Read the model definition and answer for the solid it produces. Units are mm, in the model's axes. A direction names the side the tool comes from. Give positions to 0.01 mm unless a question says otherwise; leave off trailing zeros. Loops run counter-clockwise (first coordinate to the right, second up) from the corner with the lowest first, then second, coordinate; pieces in that order, holes last. Notation, with made-up numbers: (2.25, -10.5) - (51.25, -10.5) arc R16 ccw to (51.25, 20.5) - close; hole circle Ø2 at (-35.75, 76). An arc over 180 degrees is marked (long way). Use a Markdown table: item, result. Add a question column.
Item 1: A cutting plane is placed at C-C (x = 0). Determine the outline of the cut face in (y, z).
Item 2: For a pull along Z with two mould halves and no side action, classify faces 1 (the face through (-4, 15, -1)), 2 (the face through (3.3, 5.1, 2.2)), 3 (the face through (3.417, 4.558, 0.759)) as +Z half, -Z half, draft (parallel to the pull), parting line (faces both ways), or undercut.
Item 3: Each of these flat-tipped pins is pushed along its axis until it touches: P1, Ø3, axis at x = -1.5, y = 15.5, coming from the +Z side; P2, Ø1, axis at x = 3, y = 16, coming from the +Z side; P3, Ø1.5, axis at x = 4, y = 17, coming from the +Z side. Where does it stop, or does it pass through?
Item 4: A cutting plane is placed at A-A (y = 13.25). Determine the outline of the cut face in (x, z).
Item 5: Consider probe 1 along Z at (x, y) = (-1, 12.75); probe 2 along X at (y, z) = (11, -0.5); probe 3 along Z at (x, y) = (-4, 16.75). Determine where each line is inside the solid, lowest interval first. Write a range as [from, to].
Item 6: Which of the six approach directions +Z, -Z, +X, -X, +Y, -Y give full straight-line access (tool end or side, diameter ignored) to faces 4 (the face through (0.09, 16.16, -4.75)), 5 (the face through (2, 4, 2)), 6 (the face through (-0.09, 16.16, 4.75)), 7 (the face through (0, 14, -3))?
Item 7: A cutting plane is placed at B-B (z = 0). Determine the outline of the cut face in (x, y), plus the area to 3 significant figures.
Item 8: A cutting plane is placed at D-D (y = 6). Determine the outline of the cut face in (x, z).
from build123d import *

# Parameters (mm, degrees)
ENL_V_MAT_EXTRU_1_REACH             = 23.308
ESQUISSE2_W                         = 2
ESQUISSE2_H                         = 8
ENL_V_MAT_EXTRU_1_DIRECTION_2_REACH = 23.308


with BuildPart() as part:
    # Esquisse1 → Révolution1 (revolve)
    with BuildSketch(Plane.XY, mode=Mode.PRIVATE) as r_volution1_sk:
        with BuildLine():
            Line((0, 0), (-2.5, 0))
            Line((-2.5, 0), (-2.5, 4))
            Line((-2.5, 4), (-3.5, 4))
            Line((-3.5, 4), (-3.5, 5.1))
            Line((-3.5, 5.1), (-5, 5.1))
            Line((-5, 5.1), (-5, 12.1))
            Line((-5, 12.1), (-4.75, 12.1))
            Line((-4.75, 12.1), (-4.75, 20.1))
            Line((-4.75, 20.1), (-4.55, 20.1))
            Line((-4.55, 20.1), (-3, 16.1))
            Line((-3, 16.1), (-3, 12.1))
            ThreePointArc((-3, 12.1), (-2.121320344, 9.978679656), (0, 9.1))
            Line((0, 9.1), (0, 0))
        make_face()
    revolve(r_volution1_sk.sketch.rotate(Axis((0, -1.292585524, 0), (0, 1, 0)), 270), axis=Axis((0, -1.292585524, 0), (0, 1, 0)))

    # Esquisse2 → Enlèv. mat.-Extru.1 (cut, up to next)
    with BuildSketch(Plane(origin=(0, 0, 0), x_dir=(0, 0, -1), z_dir=(1, 0, 0)), mode=Mode.PRIVATE) as enl_v_mat_extru_1_sk1:
        with Locations((0, 16.1)):
            Rectangle(ESQUISSE2_W, ESQUISSE2_H)
    enl_v_mat_extru_1_tool1 = extrude(enl_v_mat_extru_1_sk1.sketch, amount=-ENL_V_MAT_EXTRU_1_REACH, mode=Mode.PRIVATE) & part.part
    add(enl_v_mat_extru_1_tool1.solids().sort_by_distance((0, 16.1, 0))[0], mode=Mode.SUBTRACT)

    # Esquisse2 → Enlèv. mat.-Extru.1 direction 2 (cut, up to next)
    with BuildSketch(Plane(origin=(0, 0, 0), x_dir=(0, 0, -1), z_dir=(1, 0, 0)), mode=Mode.PRIVATE) as enl_v_mat_extru_1_direction_2_sk1:
        with Locations((0, 16.1)):
            Rectangle(ESQUISSE2_W, ESQUISSE2_H)
    enl_v_mat_extru_1_direction_2_tool1 = extrude(enl_v_mat_extru_1_direction_2_sk1.sketch, amount=ENL_V_MAT_EXTRU_1_DIRECTION_2_REACH, mode=Mode.PRIVATE) & part.part
    add(enl_v_mat_extru_1_direction_2_tool1.solids().sort_by_distance((0, 16.1, 0))[0], mode=Mode.SUBTRACT)


solid = part.part
Geometry says:
| question | item | result |
|---|---|---|
| 1 | outline | (0, -2.5) - (4, -2.5) - (4, -3.5) - (5.1, -3.5) - (5.1, -5) - (12.1, -5) - (12.1, -4.75) - (20.1, -4.75) - (20.1, -4.55) - (16.1, -3) - (12.1, -3) arc R3 cw to (12.1, 3) - (16.1, 3) - (20.1, 4.55) - (20.1, 4.75) - (12.1, 4.75) - (12.1, 5) - (5.1, 5) - (5.1, 3.5) - (4, 3.5) - (4, 2.5) - (0, 2.5) - close |
| 2 | face 1 | undercut |
| 2 | face 2 | draft |
| 2 | face 3 | parting line |
| 3 | P1 | z = 4.75 |
| 3 | P2 | z = 4.04 |
| 3 | P3 | z = 3.46 |
| 4 | outline | (-4.64, -1) arc R4.75 ccw to (4.64, -1) - (2.83, -1) arc R3 cw to (-2.83, -1) - close; (-4.64, 1) - (-2.83, 1) arc R3 cw to (2.83, 1) - (4.64, 1) arc R4.75 ccw to start |
| 5 | probe 1 | [-4.64, -2.83], [2.83, 4.64] |
| 5 | probe 2 | [-4.97, -2.75], [2.75, 4.97] |
| 5 | probe 3 | [-2.56, -1], [1, 2.56] |
| 6 | face 4 | -Z, +Y |
| 6 | face 5 | -Y |
| 6 | face 6 | +Z, +Y |
| 6 | face 7 | +Y |
| 7 | outline | (-5, 5.1) - (-3.5, 5.1) - (-3.5, 4) - (-2.5, 4) - (-2.5, 0) - (2.5, 0) - (2.5, 4) - (3.5, 4) - (3.5, 5.1) - (5, 5.1) - (5, 12.1) - (3, 12.1) arc R3 cw to (-3, 12.1) - (-5, 12.1) - close |
| 7 | area | 83.6 mm² |
| 8 | outline | circle Ø10 at (0, 0) |
